Autodesk Inventor part; units mm, degrees
ref_plane "YZ Plane" through (0, 0, 0) normal (1, 0, 0) x (0, 1, 0)
ref_plane "XZ Plane" through (0, 0, 0) normal (0, 1, 0) x (-1, 0, 0)
ref_plane "XY Plane" through (0, 0, 0) normal (0, 0, 1) x (1, 0, 0)
sketch "Sketch1" plane through (0, 0, 0) normal (0, 1, 0) x (-1, 0, 0)
  circle A0 centre (0, 0) radius 32.5
  circle A1 centre (0, 0) radius 35.5
  dimension "d0" = 65
  dimension "d1" = 71
extrude "Extrusion1" add sketch "Sketch1" along normal blind 8
extrude "Extrusion2" add sketch "Sketch1" along normal blind 3 contours A0
fillet "Fillet1" radius 2 2 edges at (35.5, 0, 0) (32.5, 3, 0)
fillet "Fillet2" radius 1.5 2 edges at (32.5, 8, 0) (35.5, 8, 0)
properties part number "Orchid Coaster V2"
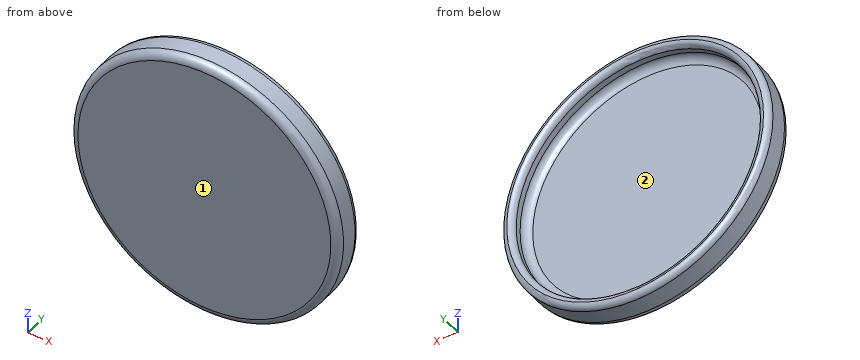
Geometry check sheet. Reference: the model listing, model coordinates, mm. Face numbers are marked on the shaded views. Coordinates: 2 decimals unless noted, no trailing zeros.
Item 1: Thickness scan on line 1 (Z direction, x = 0, y = 5.65); line 2 (Y direction, x = -29, z = -9); line 3 (Z direction, x = -9, y = 6.25). Record the ranges inside material, lowest first.
Item 2: Release check for a two-part mould opening along X. For the marked faces 1 and 2 record: released by +X, released by -X, zero draft, split by the parting line, or undercut.
Item 3: Go/stop test with flat-tipped pins: pin 1 Ø3 at (y, z) = (2.5, 6) entering from -X; pin 2 Ø2 at (x, z) = (-5.5, 9.5) entering from -Y; pin 3 Ø1.5 at (x, z) = (2, -13.5) entering from +Y; pin 4 Ø1 at (x, y) = (9.5, 1.5) entering from +Z. Record where each tip stops, or that it passes through.
Check result:
1. line 1: z = -35.5 to -32.5, 32.5 to 35.5
1. line 2: y = 0 to 3
1. line 3: z = -34.34 to -31.23, 31.23 to 34.34
2. face 1: zero draft
2. face 2: undercut
3. pin 1: stops at x = -35.21
3. pin 2: stops at y = 0
3. pin 3: stops at y = 3
3. pin 4: stops at z = 34.31
